```python
from build123d import *

# Parameters (mm, degrees)
BOSS_EXTRUDE1_DEPTH                        = 42
FILLET1_R                                  = 5
CBORE_FOR_M12_HEX_HEAD_BOLT2_OUTLINE_R     = 7.5
CBORE_FOR_M12_HEX_HEAD_BOLT2_DEPTH         = 23
CBORE_START                                = 15.5
CBORE_FOR_M12_HEX_HEAD_BOLT2_2_OUTLINE_R   = 11.8925
CBORE_FOR_M12_HEX_HEAD_BOLT2_2_OUTLINE_R_2 = 7.5
CBORE_FOR_M12_HEX_HEAD_BOLT2_2_DEPTH       = 7.5


# Read off the part's stored shape, not the designer's step: CBORE for M12 Hex Head Bolt2
with BuildPart() as part:
    # Sketch1 → Boss-Extrude1 (new body)
    with BuildSketch(Plane.XY):
        with BuildLine():
            Line((0, 0), (-95.5, 0))
            Line((-95.5, 0), (-95.5, 23))
            Line((-95.5, 23), (-62.057478344, 23))
            Line((-62.057478344, 23), (-56.445279918, 62.932866755))
            ThreePointArc((-56.445279918, 62.932866755), (-37.395364652, 98.018446073), (0, 112))
            Line((0, 112), (0, 96))
            ThreePointArc((0, 96), (-41, 55), (0, 14))
            Line((0, 14), (0, 0))
        make_face()
    boss_extrude1 = extrude(amount=BOSS_EXTRUDE1_DEPTH)

    # Mirror1: Boss-Extrude1 across plane
    add(boss_extrude1.mirror(Plane(origin=(0, 112, 42), x_dir=(0, 0, 1), z_dir=(-1, 0, 0))))

    # Fillet1
    fillet1_edges = [part.edges().sort_by_distance(p)[0] for p in [
        (0, 112, 0),
        (-95.5, 23, 21),
        (-62.057478344, 23, 21),
        (0, 112, 42),
        (-59.251379131, 42.966433377, 42),
        (95.5, 11.5, 42),
        (-78.778739172, 23, 42),
        (78.778739172, 23, 42),
        (95.5, 23, 21),
        (59.251379131, 42.966433377, 42),
        (62.057478344, 23, 21),
        (59.251379131, 42.966433377, 0),
        (78.778739172, 23, 0),
        (-95.5, 11.5, 42),
        (95.5, 11.5, 0),
        (-95.5, 11.5, 0),
        (-78.778739172, 23, 0),
        (-59.251379131, 42.966433377, 0),
    ]]
    fillet(fillet1_edges, radius=FILLET1_R)

    # CBORE for M12 Hex Head Bolt2 outline → CBORE for M12 Hex Head Bolt2 (cut)
    with BuildSketch(Plane(origin=(0, 0, 0), x_dir=(1, 0, 0), z_dir=(0, 1, 0))):
        with Locations((75, -21)):
            Circle(CBORE_FOR_M12_HEX_HEAD_BOLT2_OUTLINE_R)
        with Locations((-75, -20.635902385)):
            Circle(CBORE_FOR_M12_HEX_HEAD_BOLT2_OUTLINE_R)
    extrude(amount=CBORE_FOR_M12_HEX_HEAD_BOLT2_DEPTH, mode=Mode.SUBTRACT)

    # CBORE for M12 Hex Head Bolt2 2 outline → CBORE for M12 Hex Head Bolt2 2 (cut)
    # profile 1 of 2: a face of its own
    with BuildSketch(Plane(origin=(0, 0, 0), x_dir=(1, 0, 0), z_dir=(0, 1, 0)).offset(CBORE_START)):
        with Locations((75, -21)):
            Circle(CBORE_FOR_M12_HEX_HEAD_BOLT2_2_OUTLINE_R)
        with Locations((75, -21)):
            Circle(CBORE_FOR_M12_HEX_HEAD_BOLT2_2_OUTLINE_R_2, mode=Mode.SUBTRACT)
    # profile 2 of 2: a face of its own
    with BuildSketch(Plane(origin=(0, 0, 0), x_dir=(1, 0, 0), z_dir=(0, 1, 0)).offset(CBORE_START)):
        with Locations((-75, -20.635902385)):
            Circle(CBORE_FOR_M12_HEX_HEAD_BOLT2_2_OUTLINE_R)
        with Locations((-75, -20.635902385)):
            Circle(CBORE_FOR_M12_HEX_HEAD_BOLT2_2_OUTLINE_R_2, mode=Mode.SUBTRACT)
    extrude(amount=CBORE_FOR_M12_HEX_HEAD_BOLT2_2_DEPTH, mode=Mode.SUBTRACT)


solid = part.part
```
Input: part model. Units: mm. Frame: model coordinates. A direction names the side the tool comes from. Give positions to 0.01 mm unless a question says otherwise; leave off trailing zeros. Order: outer loops, then holes, each group sorted by start corner. A loop starts at its lowest first (then second) coordinate and runs counter-clockwise, first axis right, second up. Notation, with made-up numbers: M 2,3.5 L 53,3.5 A8 cw 53,15.5 Z; hole C -11.5,-28 d7. An arc over 180 degrees is marked long. One line per question, with ' | ' between items. Start each with the question number.
1. Material intervals for probe 1 along Y at (x, z) = (-1.5, 28); probe 2 along Z at (x, y) = (-75, 10.5); probe 3 along Z at (x, y) = (75, 17.75), sorted ascending. Write a range as [from, to].
2. Access query for faces 5 (the face through (-78, 21, 41)), 6 (the face through (-78, 22, 2)), 7 (the face through (78, 21, 41)), 8 (the face through (-87, 23, 24)), 9 (the face through (78, 22, 2)). Directions: +Z, -Z, +X, -X, +Y, -Y. A direction counts if a zero-diameter tool reaches every point of the face in a straight line with its end or side. Return the directions, or none.
3. Section query B-B (z = 24). Count the separate pieces of the cut face and the enclosed holes in it, and give its area (3 significant figures).
4. First-contact query: pin 1 Ø10 at (y, z) = (60.5, 37) entering from -X; pin 2 Ø3 at (y, z) = (49.5, 28) entering from -X; pin 3 Ø19.5 at (x, z) = (-75, 20.64) entering from +Y (3 decimals). Flat tips, straight axial feed; report the tip coordinate or a pass-through.
5. Section query A-A (x = 75). Return the cut outline in (y, z).
6. Pull-direction query (Z, two-part tool) for faces 1 (the face through (-94, 21.57, 21.22)), 2 (the face through (63.12, 19.2, 20.48)), 3 (the face through (-57.5, 44.66, 40.57)), 4 (the face through (-86.88, 19.2, 20.11)); classes: released by +Z, released by -Z, zero draft, split by the parting line, or undercut.
Here are the results:
1) probe 1: [0, 14.03], [95.97, 111.98] | probe 2: [0, 13.14], [28.14, 42] | probe 3: [0, 9.11], [32.89, 42]
2) face 5: +Z, -X, +Y | face 6: -Z, -X, +Y | face 7: +Z, +X, +Y | face 8: +Z, -Z, -X, +Y | face 9: -Z, +X, +Y
3) separate pieces: 3 | enclosed holes: 1 | area: 7,280 mm²
4) pin 1: x = -57.49 | pin 2: x = -58.54 | pin 3: y = 23.135
5) outline: M 0,0 L 18,0 A5 ccw 23,5 L 23,9.11 L 15.5,9.11 L 15.5,13.5 L 0,13.5 Z; M 0,28.5 L 15.5,28.5 L 15.5,32.89 L 23,32.89 L 23,37 A5 ccw 18,42 L 0,42 Z
6) face 1: zero draft | face 2: undercut | face 3: released by +Z | face 4: undercut
